For this review, use the dimensioned drawing (mm, ordinates from the lowest corner) and the shaded views. Give positions to 0.01 mm unless a question says otherwise; leave off trailing zeros. Loops run counter-clockwise (first coordinate to the right, second up) from the corner with the lowest first, then second, coordinate; pieces in that order, holes last. Notation, with made-up numbers: (72.25, 51.25) - (108.25, 51.25) arc R7 cw to (108.25, 63.25) - close; hole circle Ø1 at (30, 37). An arc over 180 degrees is marked (long way). Put each result on its own line as item: value.
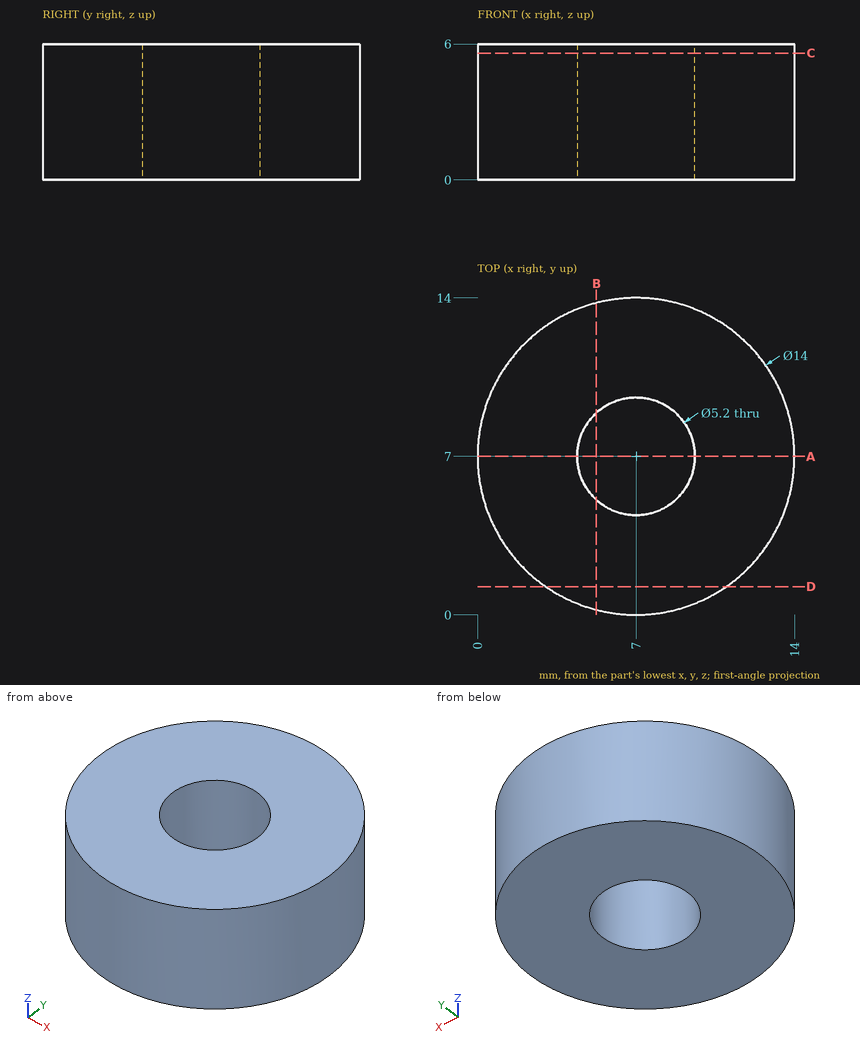
1) Take a section at C-C on z = 5.6. State the section outline as (x, y) points.
Geometry check:
outline: circle Ø14 at (7, 7); hole circle Ø5.2 at (7, 7)
2) Take a section at A-A on y = 7. State the section outline as (x, z) points.
Geometry check:
outline: (0, 0) - (4.4, 0) - (4.4, 6) - (0, 6) - close; (9.6, 0) - (14, 0) - (14, 6) - (9.6, 6) - close
3) Wall thickness on line 1 (Y direction, x = 7, z = 3.2); line 2 (X direction, y = 5.5, z = 0.7); line 3 (Y direction, x = 2, z = 1.1): over which ranges is each line inside the solid? List them lowest first.
Geometry check:
line 1: y = 0 to 4.4, 9.6 to 14
line 2: x = 0.16 to 4.88, 9.12 to 13.84
line 3: y = 2.1 to 11.9
4) Take a section at B-B on x = 5.25. State the section outline as (y, z) points, and give its area (3 significant figures).
Geometry check:
outline: (0.22, 0) - (5.08, 0) - (5.08, 6) - (0.22, 6) - close; (8.92, 0) - (13.78, 0) - (13.78, 6) - (8.92, 6) - close
area: 58.3 mm²
5) Take a section at D-D on y = 1.25. State the section outline as (x, z) points.
Geometry check:
outline: (3.01, 0) - (10.99, 0) - (10.99, 6) - (3.01, 6) - close
6) Insertion check: pin 1 Ø1.5 at (x, z) = (12.5, 4) entering from +Y; pin 2 Ø3 at (x, y) = (11.5, 3.5) entering from -Z. Each pin has a flat end and moves straight along its axis. Give the tip position at first contact, or say it passes through.
Geometry check:
pin 1: stops at y = 12.14
pin 2: stops at z = 0
